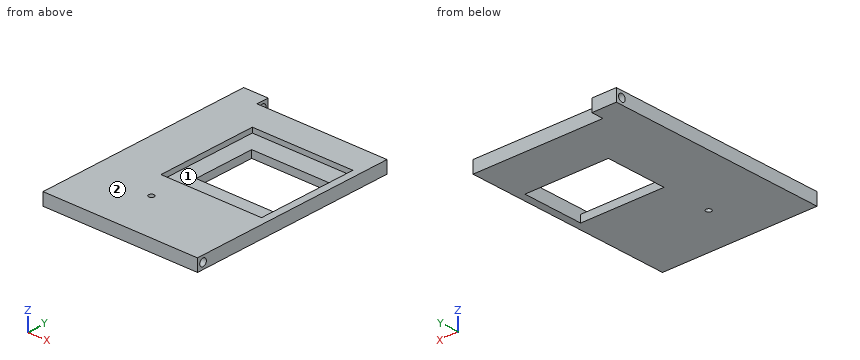
```python
from build123d import *

# Parameters (mm, degrees)
BOSS_EXTRU_1_DEPTH       = 5
ESQUISSE8_W              = 34
ESQUISSE8_H              = 25
ENL_V_MAT_EXTRU_6_DEPTH  = 5
ENL_V_START              = -5
ESQUISSE9_W              = 41
ESQUISSE9_H              = 41
ENL_V_MAT_EXTRU_7_DEPTH  = 2
ENL_V_MAT_EXTRU_8_REACH  = 111.973
ESQUISSE10_R             = 1.5
ESQUISSE12_R             = 1.5
ENL_V_MAT_EXTRU_10_DEPTH = 15
ENL_V_MAT_EXTRU_11_REACH = 111.973
ESQUISSE6_R              = 1.1


with BuildPart() as part:
    # Esquisse1 → Boss.-Extru.1 (new body)
    with BuildSketch(Plane.XY):
        Polygon((0, 0), (0, 85), (0, 90), (10, 90), (10, 85), (63, 85), (63, 0), align=None)
    extrude(amount=BOSS_EXTRU_1_DEPTH)

    # Esquisse8 → Enlèv. mat.-Extru.6 (cut)
    with BuildSketch(Plane(origin=(0, 0, 0), x_dir=(-1, 0, 0), z_dir=(0, 0, -1))):
        with Locations((-43, 52.5)):
            Rectangle(ESQUISSE8_W, ESQUISSE8_H)
    extrude(amount=-ENL_V_MAT_EXTRU_6_DEPTH, mode=Mode.SUBTRACT)

    # Esquisse9 → Enlèv. mat.-Extru.7 (cut)
    with BuildSketch(Plane(origin=(0, 0, 0), x_dir=(-1, 0, 0), z_dir=(0, 0, -1)).offset(ENL_V_START)):
        with Locations((-39.5, 52.5)):
            Rectangle(ESQUISSE9_W, ESQUISSE9_H)
    extrude(amount=ENL_V_MAT_EXTRU_7_DEPTH, mode=Mode.SUBTRACT)

    # Esquisse10 → Enlèv. mat.-Extru.8 (cut, up to next)
    with BuildSketch(Plane.ZY, mode=Mode.PRIVATE) as enl_v_mat_extru_8_sk1:
        with Locations((2.5, 87.5)):
            Circle(ESQUISSE10_R)
    enl_v_mat_extru_8_tool1 = extrude(enl_v_mat_extru_8_sk1.sketch, amount=-ENL_V_MAT_EXTRU_8_REACH, mode=Mode.PRIVATE) & part.part
    add(enl_v_mat_extru_8_tool1.solids().sort_by_distance((0, 87.5, 2.5))[0], mode=Mode.SUBTRACT)

    # Esquisse12 → Enlèv. mat.-Extru.10 (cut)
    with BuildSketch(Plane(origin=(63, 0, 0), x_dir=(0, 0, -1), z_dir=(1, 0, 0))):
        with Locations((-2.5, 2.5)):
            Circle(ESQUISSE12_R)
    extrude(amount=-ENL_V_MAT_EXTRU_10_DEPTH, mode=Mode.SUBTRACT)

    # Esquisse6 → Enlèv. mat.-Extru.11 (cut, up to next)
    with BuildSketch(Plane(origin=(0, 0, 0), x_dir=(-1, 0, 0), z_dir=(0, 0, -1)), mode=Mode.PRIVATE) as enl_v_mat_extru_11_sk1:
        with Locations((-26, 20)):
            Circle(ESQUISSE6_R)
    enl_v_mat_extru_11_tool1 = extrude(enl_v_mat_extru_11_sk1.sketch, amount=-ENL_V_MAT_EXTRU_11_REACH, mode=Mode.PRIVATE) & part.part
    add(enl_v_mat_extru_11_tool1.solids().sort_by_distance((26, 20, 0))[0], mode=Mode.SUBTRACT)


solid = part.part
```
Geometry: final body of the model. Coordinates: model frame, mm. Face numbers are marked on the shaded views. Round coordinates to 2 decimals unless told otherwise and drop trailing zeros. Write each loop counter-clockwise with the first axis right and the second up, starting at its lowest first coordinate (ties: lowest second). Pieces come first, ordered by that corner, then holes. Notation, with made-up numbers: (-28.5, 77) -> (23.5, 77) arc R19 ccw to (23.5, 86) -> close; hole circle Ø8 at (-2.5, -13.5). An arc over 180 degrees is marked (long way). Return JSON: item names as keys, results as strings.
Q1. Mould query, pull axis X, two halves, no side actions, for the marked faces 1 and 2. Classes: +X half, -X half, draft (parallel to the pull), parting line (faces both ways), or undercut.
From the geometry:
{"face 1": "undercut", "face 2": "draft"}
Q2. Section C-C on x = 28. Return the cut outline in (y, z).
From the geometry:
{"outline": "(0, 0) -> (40, 0) -> (40, 3) -> (32, 3) -> (32, 5) -> (0, 5) -> close; (65, 0) -> (85, 0) -> (85, 5) -> (73, 5) -> (73, 3) -> (65, 3) -> close"}
Q3. Ray query, line 1 (X direction, y = 45.5, z = 2.15); line 2 (X direction, y = 38.5, z = 4); line 3 (Y direction, x = 3.5, z = 2.75). Return the intervals inside material, ascending.
From the geometry:
{"line 1": "0 to 26, 60 to 63", "line 2": "0 to 19, 60 to 63", "line 3": "0 to 86.02, 88.98 to 90"}
Q4. Section B-B on y = 87.5. Return the cut outline in (x, z), and give its area (3 significant figures).
From the geometry:
{"outline": "(0, 0) -> (10, 0) -> (10, 1) -> (0, 1) -> close; (0, 4) -> (10, 4) -> (10, 5) -> (0, 5) -> close", "area": "20.0 mm2"}
Q5. First-contact query: pin 1 Ø4 at (x, y) = (52.5, 22.5) entering from -Z; pin 2 Ø2 at (x, y) = (26, 20) entering from +Z; pin 3 Ø1 at (x, z) = (29.5, 3.5) entering from +Y; pin 4 Ø2.5 at (y, z) = (86.5, 1.5) entering from +X. Flat tips, straight axial feed; report the tip coordinate or a pass-through.
From the geometry:
{"pin 1": "z = 0", "pin 2": "through", "pin 3": "y = 85", "pin 4": "x = 10"}
Q6. Section A-A on x = 55.5. Return the cut outline in (y, z), and give its area (3 significant figures).
From the geometry:
{"outline": "(0, 0) -> (40, 0) -> (40, 3) -> (32, 3) -> (32, 5) -> (0, 5) -> close; (65, 0) -> (85, 0) -> (85, 5) -> (73, 5) -> (73, 3) -> (65, 3) -> close; hole circle Ø3 at (2.5, 2.5)", "area": "261 mm2"}
Q7. Section D-D on y = 2.5. Return the cut outline in (x, z).
From the geometry:
{"outline": "(0, 0) -> (63, 0) -> (63, 1) -> (48, 1) -> (48, 4) -> (63, 4) -> (63, 5) -> (0, 5) -> close"}
